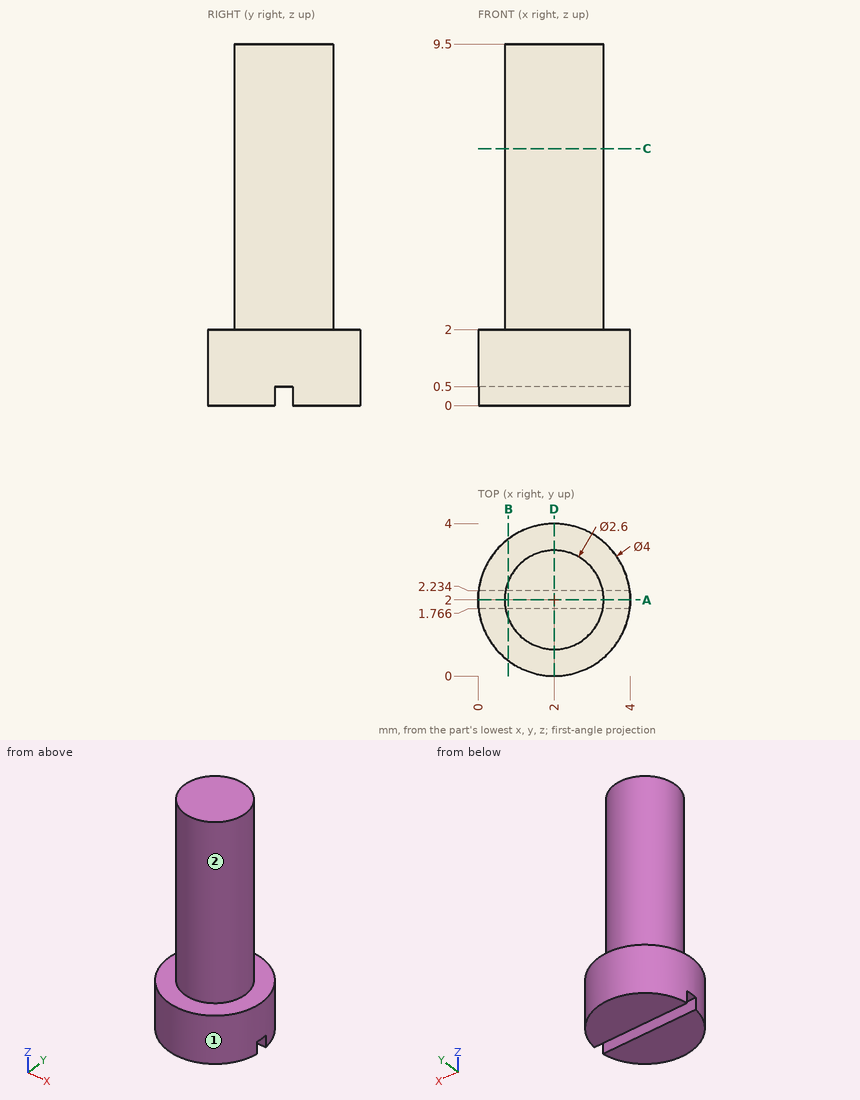
Input: dimensioned drawing with shaded views. Units: mm. Origin: part minimum x, y, z. A direction names the side the tool comes from. Coordinates: 2 decimals unless noted, no trailing zeros. Loops run counter-clockwise (first coordinate to the right, second up) from the corner with the lowest first, then second, coordinate; pieces in that order, holes last. Notation, with made-up numbers: M 30.5,83.25 L 80.5,83.25 A30 ccw 80.5,117.25 Z; hole C 7.25,6 d9. An arc over 180 degrees is marked long. One line per item, written item: value.
(1) Section B-B (x = 0.8). Output: boundary loops of the cut face in (y, z).
Filled in:
outline: M 0.4,0 L 1.77,0 L 1.77,0.5 L 2.23,0.5 L 2.23,0 L 3.6,0 L 3.6,2 L 2.5,2 L 2.5,9.5 L 1.5,9.5 L 1.5,2 L 0.4,2 Z
(2) Line query: line 1 along Z through (x, y) = (0.55, 3.15); line 2 along Z through (x, y) = (2.9, 2.05); line 3 along Y through (x, z) = (1.9, 5.5). Output: solid intervals per line, ascending. Write a range as from..to.
Filled in:
line 1: 0..2
line 2: 0.5..9.5
line 3: 0.7..3.3
(3) Section C-C (z = 6.75). Output: boundary loops of the cut face in (x, y).
Filled in:
outline: C 2,2 d2.6
(4) Section A-A (y = 2). Output: boundary loops of the cut face in (x, z).
Filled in:
outline: M 0,0.5 L 4,0.5 L 4,2 L 3.3,2 L 3.3,9.5 L 0.7,9.5 L 0.7,2 L 0,2 Z
(5) Pin query (flat end, axial travel): pin 1 (2 mm diameter, centred on x = 1.5, z = 3.5, fed in from -Y); pin 2 (1 mm diameter, centred on y = 2.5, z = 6.5, fed in from -X). Return the tip coordinate at first contact, or that it passes through.
Filled in:
pin 1: y = 0.7
pin 2: x = 0.7
(6) Reachability of the marked faces 1 and 2 from +Z, -Z, +X, -X, +Y, -Y: full face, straight path, thin tool, end or side. Return the list, or none.
Filled in:
face 1: +Z, -Z
face 2: +Z
(7) Section D-D (x = 2). Output: boundary loops of the cut face in (y, z).
Filled in:
outline: M 0,0 L 1.77,0 L 1.77,0.5 L 2.23,0.5 L 2.23,0 L 4,0 L 4,2 L 3.3,2 L 3.3,9.5 L 0.7,9.5 L 0.7,2 L 0,2 Z
